Autodesk Inventor part; units mm, degrees
ref_plane "YZ Plane" through (0, 0, 0) normal (1, 0, 0) x (0, 1, 0)
ref_plane "XZ Plane" through (0, 0, 0) normal (0, 1, 0) x (-1, 0, 0)
ref_plane "XY Plane" through (0, 0, 0) normal (0, 0, 1) x (1, 0, 0)
sketch "Sketch1" plane through (0, 0, 0) normal (0, 0, 1) x (1, 0, 0)
  line L0 (80, 0) -> (150, 0)
  line L1 (230, 10) -> (230, 100)
  line L2 (230, 100) -> (0, 100)
  line L3 (0, 100) -> (0, 10)
  line L4 (80, 0) -> (150, 0)
  line L5 (150, 0) -> (150, 10)
  line L6 (80, 10) -> (80, 0)
  line L7 (80, 10) -> (0, 10)
  line L8 (150, 10) -> (230, 10)
  dimension "d9" = 230
  dimension "d13" = 100
  dimension "d14" = 10
extrude "Extrusion1" add sketch "Sketch1" along normal blind 10
properties part number "front"
Geometry: final body of the model. Coordinates: model frame, mm. A direction names the side the tool comes from. Coordinates: 2 decimals unless noted, no trailing zeros. Write each loop counter-clockwise with the first axis right and the second up, starting at its lowest first coordinate (ties: lowest second). Pieces come first, ordered by that corner, then holes. Notation, with made-up numbers: M -13,12 L 13,12 A28 ccw 13,45 Z; hole C 46,62.25 d7. An arc over 180 degrees is marked long. Use CSV: the item, a comma, the result in double quotes. Start each with the question number.
1. First-contact query: P1, Ø4, axis at y = 10.5, z = 4.5, coming from the -X side; P2, Ø5, axis at y = 4.5, z = 3.5, coming from the +X side; P3, Ø3, axis at y = 6, z = 7, coming from the -X side; P4, Ø3, axis at x = 175.5, z = 4, coming from the -Y side. Flat tips, straight axial feed; report the tip coordinate or a pass-through.
2. Reachability of faces 4 (the face through (113, 51, 10)), 5 (the face through (189, 10, 5)), 6 (the face through (41, 10, 5)) from +Z, -Z, +X, -X, +Y, -Y: full face, straight path, thin tool, end or side. Return the list, or none.
3. Cut plane A-A on z = 4.25. Return the cut outline in (x, y).
4. Mould query, pull axis X, two halves, no side actions, for faces 1 (the face through (80, 5, 5)), 2 (the face through (150, 5, 5)), 3 (the face through (113, 51, 0)). Classes: pulls with the +X half, pulls with the -X half, needs draft (parallel to the pull), parting line crosses it, or undercut.
5. Cut plane B-B on x = 188.5. Return the cut outline in (y, z), plus the area to 3 significant figures.
6. Ray query, probe 1 along Y at (x, z) = (33, 9). Return the intervals inside material, ascending.
Entries:
1,P1,"x = 0"
1,P2,"x = 150"
1,P3,"x = 80"
1,P4,"y = 10"
2,face 4,"+Z, +X, -X, +Y, -Y"
2,face 5,"+Z, -Z, +X, -Y"
2,face 6,"+Z, -Z, -X, -Y"
3,outline,"M 0,10 L 80,10 L 80,0 L 150,0 L 150,10 L 230,10 L 230,100 L 0,100 Z"
4,face 1,"pulls with the -X half"
4,face 2,"pulls with the +X half"
4,face 3,"needs draft"
5,outline,"M 10,0 L 100,0 L 100,10 L 10,10 Z"
5,area,"900 mm²"
6,probe 1,"10 to 100"
